Read the model definition and answer for the solid it produces. Units are mm, in the model's axes. Face numbers are marked on the shaded views. Round coordinates to 2 decimals unless told otherwise and drop trailing zeros. Loops run counter-clockwise (first coordinate to the right, second up) from the corner with the lowest first, then second, coordinate; pieces in that order, holes last. Notation, with made-up numbers: M -29.5,67 L 29.5,67 A36 ccw 29.5,106 Z; hole C 84.5,14 d11. An arc over 180 degrees is marked long. Write each question's results on one line, items separated by ' | '.
Autodesk Inventor part; units mm, degrees
ref_plane "Plano de trabajo1" through (-26.5, -52.5, 0.96) normal (0, 0, 1) x (0, 1, 0)
ref_plane "Plano de trabajo2" through (-13.75, 27.5, -0.5) normal (-1, 0, 0) x (0, 0, 1)
ref_plane "YZ Plane" through (0, 0, 0) normal (1, 0, 0) x (0, 1, 0)
sketch "Boceto1" plane through (0, 0, 0) normal (0, 0, 1) x (1, 0, 0)
  line L0 (0, 0) -> (51, 0)
  line L1 (51, 0) -> (51, 27.5)
  line L2 (51, 27.5) -> (0, 27.5)
  line L3 (-0.5, 1) -> (51, 1)
  line L4 (0, 26.5) -> (51, 26.5)
  line L5 (0, 27.5) -> (-27.5, 27.5)
  line L6 (-27.5, 27.5) -> (-27.5, -52.5)
  line L7 (-27.5, -52.5) -> (0, -52.5)
  line L8 (0, -52.5) -> (0, 0)
  line L9 (0, 26.5) -> (-26.5, 26.5)
  line L10 (-0.5, 1) -> (-1, 1)
  line L11 (-1, 1) -> (-1, -52.5)
  line L12 (-26.5, 26.5) -> (-26.5, -52.5)
  dimension "d0" = 51
  dimension "d1" = 27.5
  dimension "d2" = 1
  dimension "d3" = 1
  dimension "d4" = 27.5
  dimension "d5" = 0.5
  dimension "d6" = 1
  dimension "d7" = 1
  dimension "d8" = 80
extrude "Extrusión1" add sketch "Boceto1" against normal blind 0.5
extrude "Extrusión2" add sketch "Boceto1" along normal blind 0.96 contours L8 L7 L11 L10 L3 L1 L0 | L4 L9 L12 L7 L6 L5 L2 L1
ref_plane "Plano de trabajo1" through (-26.5, -52.5, 0.96) normal (0, 0, 1) x (0, 1, 0)
mirror "Simetría1" about plane through (-26.5, -52.5, 0.96) normal (0, 0, 1) of "Extrusión1", "Extrusión2"
sketch "Boceto2" plane through (-27.5, 27.5, 2.42) normal (0, 0, 1) x (1, 0, 0)
  line L0 (26.5, -80) -> (26.5, -26.5)
  line L1 (78.5, -27.5) -> (27.5, -27.5)
  line L2 (26.5, -27.5) -> (0, -27.5)
  line L3 (0, -80) -> (0, 0)
  line L4 (27.5, -27.5) -> (27.5, -80)
  line L5 (26.5, -29) -> (0, -29)
  line L6 (0, -29) -> (0, -27.5)
  line L7 (26.5, -29) -> (26.5, -27.5)
  line L8 (26.5, -80) -> (26.5, -26.5)
  line L9 (27.5, -27.5) -> (39.5, -27.5)
  line L10 (27.5, -27.5) -> (27.5, -36.5)
  line L11 (27.5, -36.5) -> (39.5, -27.5)
  line L12 (39.5, -27.5) -> (43.5, -27.5)
  line L13 (43.5, -27.5) -> (27.5, -39.5)
  line L14 (27.5, -39.5) -> (27.5, -36.5)
  circle A0 centre (13.25, -35) radius 5
  dimension "d13" = 1.5
  dimension "d16" = 12
  dimension "d17" = 9
  dimension "d18" = 4
  dimension "d19" = 20
  dimension "d59" = 10
  dimension "d61" = 6
extrude "Extrusión3" cut sketch "Boceto2" against normal blind 2.42 contours L5 L3 L2 L0
extrude "Extrusión4" add sketch "Boceto2" against normal blind 2.92 contours L13 L4 L11 L1
sketch "Boceto3" plane through (-27.5, -52.5, -0.5) normal (0, -1, 0) x (1, 0, 0)
  line L0 (0, 0) -> (78.5, 0)
  line L1 (78.5, 0.5) -> (1, 0.5)
  line L2 (39.5, 2.92) -> (27.5, 2.92)
  line L3 (0, 2.92) -> (0, 0)
  line L4 (27.5, 0) -> (27.5, 2.92)
  line L5 (0, 0) -> (27.5, 0)
  line L6 (27.5, 0) -> (27.5, 2.92)
  line L7 (0, 2.92) -> (26.5, 2.92)
  line L8 (27.5, 2.92) -> (26.5, 2.92)
  line L9 (26.5, 0.5) -> (26.5, 2.42)
  line L10 (26.5, 2.92) -> (26.5, 0.5)
  line L11 (26.5, 0.5) -> (1, 0.5)
  line L12 (1, 0.5) -> (1, 2.42)
  line L13 (1, 0.5) -> (1, 2.92)
  line L14 (1, 2.92) -> (0, 2.92)
extrude "Extrusión5" add sketch "Boceto3" along normal blind 25.5 contours L3 L7 L13 L12 L1 L4 L0 | L1 L9 L10 L8 L4
sketch "Boceto4" plane through (-27.5, 27.5, -0.5) normal (-1, 0, 0) x (0, 0, 1)
  line L0 (2.92, -105.5) -> (0, -105.5)
  line L1 (0.5, -29) -> (0.5, -105.5)
  line L2 (0, 0) -> (0, -105.5)
  line L3 (0.5, -105.5) -> (0, -105.5)
  line L4 (0, -39.5) -> (0, -105.5)
  line L5 (0, -105.5) -> (144.6349, -189.005)
  line L6 (2.92, -105.5) -> (0.5, -105.5)
  line L7 (0.5, -105.5) -> (145.1349, -189.005)
  line L8 (2.92, -39.5) -> (2.92, -105.5)
  line L9 (0.5, -105.5) -> (2.92, -105.5)
  line L10 (2.92, -105.5) -> (145.7399, -187.9571)
  line L11 (144.6349, -189.005) -> (145.1349, -189.005)
  line L12 (145.1349, -189.005) -> (145.7399, -187.9571)
  point P0 (0.5, -27.5)
  dimension "d26" = 30
extrude "Extrusión6" add sketch "Boceto4" against normal blind 27.5 contours L7 L11 L5 L0
ref_plane "Plano de trabajo2" through (-13.75, 27.5, -0.5) normal (-1, 0, 0) x (0, 0, 1)
extrude "Extrusión7" add sketch "Boceto4" against normal blind 1 contours L10 L12 L7 L0
mirror "Simetría2" about plane through (-13.75, 27.5, -0.5) normal (-1, 0, 0) of "Extrusión7"
sketch "Boceto5" plane through (-26.5, -78, 0) normal (0, 0.866, 0.5) x (1, 0, 0)
  line L0 (0, 0) -> (0, -167.01)
  line L1 (25.5, -167.01) -> (25.5, 0)
  line L2 (25.5, 0) -> (0, 0)
  line L3 (0, 0) -> (0, -167.01)
  line L4 (0, -167.01) -> (25.5, -167.01)
  line L5 (12.75, 0) -> (38.25, 0) construction
  circle A0 centre (12.75, -25.5) radius 10.25
  line L6 (12.75, -35.75) -> (12.75, -38.25)
  circle A1 centre (12.75, -49.25) radius 11
  line L7 (12.75, -38.25) -> (23.75, -38.25) construction
  line L8 (12.75, -60.25) -> (12.75, -62.75)
  circle A2 centre (12.75, -73.94) radius 11.19
  line L9 (12.75, -85.13) -> (12.75, -87.63)
  circle A3 centre (12.75, -99.13) radius 11.5
  line L10 (12.75, -110.63) -> (12.75, -113.13)
  circle A4 centre (12.75, -125.32) radius 12.19
  line L11 (12.75, -113.13) -> (24.94, -113.13) construction
  line L12 (12.75, -137.51) -> (12.75, -140.01)
  circle A5 centre (12.75, -152.76) radius 12.75
  line L13 (12.75, -15.25) -> (12.75, 0)
  line L14 (0, -167.01) -> (25.5, -167.01)
  line L15 (25.5, -167.01) -> (25.5, 0)
  line L16 (0, -167.01) -> (25.5, -167.01)
  line L17 (25.5, -167.01) -> (25.5, -165.51)
  line L18 (25.5, -165.51) -> (0, -165.51)
  line L19 (0, -165.51) -> (0, -167.01)
  point P0 (26.5, 39)
  dimension "d37" = 22
  dimension "d41" = 22.38
  dimension "d45" = 23
  dimension "d48" = 24.38
  dimension "d35" = 20.5
  dimension "d36" = 2.5
  dimension "d40" = 2.5
  dimension "d44" = 2.5
  dimension "d47" = 2.5
  dimension "d51" = 2.5
  dimension "d53" = 25.5
extrude "Extrusión8" cut sketch "Boceto5" against normal through all contours A5 | A4 | A0 | A3 | A1 | A2
extrude "Extrusión9" add sketch "Boceto5" along normal blind 1.21 contours L18 L1 L4 L0
extrude "Extrusión10" cut sketch "Boceto2" against normal through all contours A0
equation "\"d59\" = sensor"
equation "\"d37\" = cincuentacen"
equation "\"d41\" = dossol"
equation "\"d45\" = veintecen"
equation "\"d48\" = cincosol"
equation "\"d35\" = diezcen"
equation "\"d53\" = UnSol"
equation "\"UnSol\" = 25.5"
equation "\"diezcen\" = 20.5"
equation "\"veintecen\" = 23"
equation "\"cincuentacen\" = 22"
equation "\"dossol\" = 22.38"
equation "\"cincosol\" = 24.38"
equation "\"sensor\" = 10"
properties part number "Maquinita"
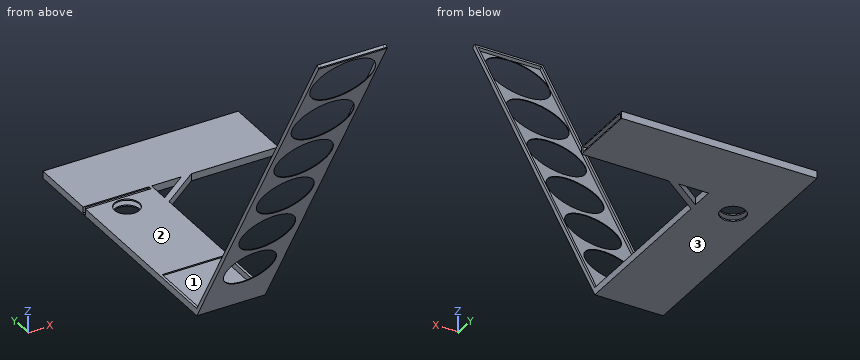
Item 1: The part is cut by section A-A (x = 8.5). Determine the outline of the cut face in (y, z) (3 decimals).
Outcome:
outline: M -5.625,-0.5 L -2.625,-0.5 L -2.625,2.42 L -5.625,2.42 Z; M 0,-0.5 L 27.5,-0.5 L 27.5,2.42 L 0,2.42 Z; hole M 1,0 L 26.5,0 L 26.5,1.92 L 1,1.92 Z
Item 2: The part is cut by section B-B (y = 6.5). Determine the outline of the cut face in (x, z).
Outcome:
outline: M -27.5,-0.5 L 51,-0.5 L 51,0 L -26.5,0 L -26.5,1.92 L 51,1.92 L 51,2.42 L -27.5,2.42 Z
Item 3: The part is cut by section C-C (y = -62). Determine the outline of the cut face in (x, z), plus the area to 3 significant figures.
Outcome:
outline: M -27.5,-0.5 L 0,-0.5 L 0,2.42 L -1,2.42 L -1,0 L -26.5,0 L -26.5,2.42 L -27.5,2.42 Z | area: 18.6 mm2
Item 4: Flat-ended cylindrical pins translate along their axes: pin 1 (1 mm diameter, centred on x = -2, z = 0.5, fed in from -Y); pin 2 (1.5 mm diameter, centred on y = -3, z = 1.5, fed in from +X); pin 3 (10 mm diameter, centred on x = -6, y = -119.5, fed in from +Z); pin 4 (16 mm diameter, centred on x = -14.25, y = -7.5, fed in from -Z). Find the tip coordinate at first contact, or state that the pin passes through.
Outcome:
pin 1: stops at y = -78.87 | pin 2: stops at x = 13 | pin 3: stops at z = 80.07 | pin 4: stops at z = -0.5
Item 5: The mould has two halves that part along Z. Classify the marked faces 1, 2 and 3: pulls with the +Z half, pulls with the -Z half, needs draft (parallel to the pull), parting line crosses it, or undercut.
Outcome:
face 1: undercut | face 2: pulls with the +Z half | face 3: pulls with the -Z half
Item 6: Straight lines are drawn through the part: line 1 (X direction, y = -7, z = 2); line 2 (Y direction, x = -14.25, z = 2.2); line 3 (Y direction, x = -14, z = 2). For each, find the intervals that lie inside material, in ascending order.
Outcome:
line 1: x = -27.5 to -19.22, -9.28 to 0, 2.67 to 6.67 | line 2: y = -79.56 to -79.27, -52.5 to -12.5, -2.5 to -1.5, 0 to 27.5 | line 3: y = -79.44 to -79.15, -52.5 to -12.49, -2.51 to -1.5, 0 to 27.5
